from build123d import *

# Parameters (mm, degrees)
SKETCH_W        = 215
SKETCH_H        = 72.5
PAD_DEPTH       = 1
SKETCH001_W     = 219
SKETCH001_H     = 76.5
PAD001_DEPTH    = 53.5
FILLET_R        = 2
FILLET001_R     = 0.5
PAD007_DEPTH    = 40
PAD008_DEPTH    = 40
PAD009_DEPTH    = 8
PAD010_DEPTH    = 8
SKETCH034_W     = 183
SKETCH034_H     = 3
POCKET011_DEPTH = 1.5
SKETCH035_R     = 2.5
POCKET012_DEPTH = 1.5
SKETCH036_R     = 1.4
SKETCH036_W     = 183
SKETCH036_H     = 3
POCKET013_DEPTH = 5
SKETCH043_W     = 6.5
SKETCH043_H     = 3
POCKET016_DEPTH = 1.5
SKETCH044_W     = 6.5
SKETCH044_H     = 3
POCKET017_DEPTH = 1.5


with BuildPart() as part:
    # Sketch → Pad (new body)
    with BuildSketch(Plane.XY):
        with BuildLine():
            Line((-112.5, 38.25), (-112.5, -38.25))
            ThreePointArc((-109.5, -41.25), (-111.62132, -40.37132), (-112.5, -38.25))
            Line((-109.5, -41.25), (109.5, -41.25))
            ThreePointArc((112.5, -38.25), (111.62132, -40.37132), (109.5, -41.25))
            Line((112.5, -38.25), (112.5, 38.25))
            ThreePointArc((109.5, 41.25), (111.62132, 40.37132), (112.5, 38.25))
            Line((109.5, 41.25), (-109.5, 41.25))
            ThreePointArc((-112.5, 38.25), (-111.62132, 40.37132), (-109.5, 41.25))
        make_face()
        Rectangle(SKETCH_W, SKETCH_H, mode=Mode.SUBTRACT)
    extrude(amount=PAD_DEPTH)

    # Sketch001 (on Face13 of Pad) → Pad001 (join)
    with BuildSketch(Plane(origin=(0, 0, 0), x_dir=(1, 0, 0), z_dir=(0, 0, -1))):
        with BuildLine():
            Line((109.5, 41.25), (-109.5, 41.25))
            ThreePointArc((-112.5, 38.25), (-111.62132, 40.37132), (-109.5, 41.25))
            Line((-112.5, 38.25), (-112.5, -38.25))
            ThreePointArc((-109.5, -41.25), (-111.62132, -40.37132), (-112.5, -38.25))
            Line((-109.5, -41.25), (109.5, -41.25))
            ThreePointArc((112.5, -38.25), (111.62132, -40.37132), (109.5, -41.25))
            Line((112.5, -38.25), (112.5, 38.25))
            ThreePointArc((109.5, 41.25), (111.62132, 40.37132), (112.5, 38.25))
        make_face()
        Rectangle(SKETCH001_W, SKETCH001_H, mode=Mode.SUBTRACT)
    extrude(amount=PAD001_DEPTH)

    # Fillet
    fillet_edges = [part.edges().sort_by_distance(p)[0] for p in [
        (112.5, 0, 1),
        (111.62132, -40.37132, 1),
        (0, -41.25, 1),
        (111.62132, 40.37132, 1),
        (0, 41.25, 1),
        (-111.62132, 40.37132, 1),
        (-112.5, 0, 1),
        (-111.62132, -40.37132, 1),
    ]]
    fillet(fillet_edges, radius=FILLET_R)

    # Fillet001
    fillet001_edges = [part.edges().sort_by_distance(p)[0] for p in [
        (0, -36.25, 1),
        (107.5, 0, 1),
        (0, 36.25, 1),
        (-107.5, 0, 1),
    ]]
    fillet(fillet001_edges, radius=FILLET001_R)

    # Sketch008 (on DatumPlane) → Pad007 (join, symmetric)
    with BuildSketch(Plane(origin=(0, 38.25, 0), x_dir=(0, 0, 1), z_dir=(1, 0, 0))):
        Polygon((-43, 0), (-33, 0), (-33, 2), align=None)
    extrude(amount=PAD007_DEPTH, both=True)

    # Sketch010 (on DatumPlane) → Pad008 (join, symmetric)
    with BuildSketch(Plane(origin=(0, -38.25, 0), x_dir=(0, 0, 1), z_dir=(-1, 0, 0))):
        Polygon((-43, 0), (-33, 0), (-33, 2), align=None)
    extrude(amount=PAD008_DEPTH, both=True)

    # Sketch012 (on DatumPlane) → Pad009 (join, symmetric)
    with BuildSketch(Plane(origin=(-109.5, 0, 0), x_dir=(0, 0, 1), z_dir=(0, 1, 0))):
        Polygon((-43, 0), (-33, 0), (-33, 0.8), align=None)
    extrude(amount=PAD009_DEPTH, both=True)

    # Sketch014 (on DatumPlane) → Pad010 (join, symmetric)
    with BuildSketch(Plane(origin=(109.5, 0, 0), x_dir=(0, 0, 1), z_dir=(0, -1, 0))):
        Polygon((-33, 0), (-43, 0), (-33, 0.8), align=None)
    extrude(amount=PAD010_DEPTH, both=True)

    # Sketch034 (on Face29 of Pad010) → Pocket011 (cut)
    with BuildSketch(Plane.XZ.offset(-38.25)):
        with Locations((0, -50)):
            Rectangle(SKETCH034_W, SKETCH034_H)
    extrude(amount=-POCKET011_DEPTH, mode=Mode.SUBTRACT)

    # Sketch035 (on Face21 of Pocket011) → Pocket012 (cut)
    with BuildSketch(Plane.XZ.offset(41.25)):
        with Locations((104.15, -48.5)):
            Circle(SKETCH035_R)
        with Locations((-104.15, -48.5)):
            Circle(SKETCH035_R)
    extrude(amount=-POCKET012_DEPTH, mode=Mode.SUBTRACT)

    # Sketch036 (on Face35 of Pocket012) → Pocket013 (cut)
    with BuildSketch(Plane.XZ.offset(39.75)):
        with Locations((104.15, -48.5)):
            Circle(SKETCH036_R)
        with Locations((-104.15, -48.5)):
            Circle(SKETCH036_R)
        with Locations((0, -50)):
            Rectangle(SKETCH036_W, SKETCH036_H)
    extrude(amount=-POCKET013_DEPTH, mode=Mode.SUBTRACT)

    # Sketch043 (on Face32 of Pocket013) → Pocket016 (cut)
    with BuildSketch(Plane(origin=(109.5, 0, 0), x_dir=(0, -1, 0), z_dir=(-1, 0, 0))):
        with Locations((0, -50)):
            Rectangle(SKETCH043_W, SKETCH043_H)
    extrude(amount=-POCKET016_DEPTH, mode=Mode.SUBTRACT)

    # Sketch044 (on Face30 of Pocket016) → Pocket017 (cut)
    with BuildSketch(Plane.YZ.offset(-109.5)):
        with Locations((0, -50)):
            Rectangle(SKETCH044_W, SKETCH044_H)
    extrude(amount=-POCKET017_DEPTH, mode=Mode.SUBTRACT)


solid = part.part
Model file for the job. Use its own axes, mm. A direction names the side the tool comes from. Give positions to 0.01 mm unless a question says otherwise; leave off trailing zeros. Loops run counter-clockwise (first coordinate to the right, second up) from the corner with the lowest first, then second, coordinate; pieces in that order, holes last.
Item 1: Drill centre lines: line 1 along X through (y, z) = (6, -30); line 2 along Z through (x, y) = (-104.15, -38.65); line 3 along Y through (x, z) = (-57.5, -25). Where is each one in solid material? Low to high.
Check values:
line 1: x = -112.5 to -109.5, 109.5 to 112.5
line 2: z = -53.5 to -49.9, -47.1 to 1
line 3: y = -41.25 to -38.25, 38.25 to 41.25
Item 2: Slice it at A-A (x = -81.5). Write the cut outline in (y, z).
Check values:
outline: (-41.25, -53.5) - (-38.25, -53.5) - (-38.25, -51.5) - (-39.75, -51.5) - (-39.75, -48.5) - (-38.25, -48.5) - (-38.25, 0) - (-36.25, 0) - (-36.25, 0.5) arc R0.5 ccw to (-36.75, 1) - (-39.25, 1) arc R2 ccw to (-41.25, -1) - close; (36.25, 0) - (38.25, 0) - (38.25, -48.5) - (39.75, -48.5) - (39.75, -51.5) - (38.25, -51.5) - (38.25, -53.5) - (41.25, -53.5) - (41.25, -1) arc R2 ccw to (39.25, 1) - (36.75, 1) arc R0.5 ccw to (36.25, 0.5) - close
Item 3: Slice it at C-C (y = -18). Write the cut outline in (x, z), plus the area to 3 significant figures.
Check values:
outline: (-112.5, -53.5) - (-109.5, -53.5) - (-109.5, 0) - (-107.5, 0) - (-107.5, 0.5) arc R0.5 ccw to (-108, 1) - (-110.5, 1) arc R2 ccw to (-112.5, -1) - close; (107.5, 0) - (109.5, 0) - (109.5, -53.5) - (112.5, -53.5) - (112.5, -1) arc R2 ccw to (110.5, 1) - (108, 1) arc R0.5 ccw to (107.5, 0.5) - close
area: 329 mm2
Item 4: Slice it at B-B (z = -20). Write the cut outline in (x, y).
Check values:
outline: (-112.5, -38.25) arc R3 ccw to (-109.5, -41.25) - (109.5, -41.25) arc R3 ccw to (112.5, -38.25) - (112.5, 38.25) arc R3 ccw to (109.5, 41.25) - (-109.5, 41.25) arc R3 ccw to (-112.5, 38.25) - close; hole (-109.5, -38.25) - (109.5, -38.25) - (109.5, 38.25) - (-109.5, 38.25) - close
Item 5: Mould opens along X. For faces 4 (the face through (-112.5, -1, -27)), 5 (the face through (109.106, -0.112, -38.07)), 6 (the face through (-2, 41.25, -27)) say: +X half, -X half, draft (parallel to the pull), parting line (faces both ways), or undercut.
Check values:
face 4: -X half
face 5: undercut
face 6: draft
Item 6: Which spindle directions (+Z, -Z, +X, -X, +Y, -Y) get a long thin tool onto all of the face, cutting with end or side? Do faces 1 (the face through (-1, 37, 0)), 2 (the face through (0.56, 37.236, -37.93)), 3 (the face through (-101.765, -40.51, -47.749)). Say none if no direction does.
Check values:
face 1: none
face 2: -Z
face 3: -Y
